Part model, mm, in its own coordinate system. A direction names the side the tool comes from. Round coordinates to 2 decimals unless told otherwise and drop trailing zeros. Write each loop counter-clockwise with the first axis right and the second up, starting at its lowest first coordinate (ties: lowest second). Pieces come first, ordered by that corner, then holes. Notation, with made-up numbers: M 63.5,84.5 L 117.5,84.5 A11 cw 117.5,89.5 Z; hole C 30,39.25 d11. An arc over 180 degrees is marked long. Answer as a JSON object with one key per item and string values. Group by question number.
1. Two-plate mould, pull along Z, no slides. Class faces 4 (the face through (-11.14, -28.26, -0.28)), 5 (the face through (-11, -27.52, 1)), 6 (the face through (-9.46, -29.85, -2.1)): +Z half, -Z half, draft (parallel to the pull), parting line (faces both ways), or undercut.
2. Band-saw the part on B-B, the plane y = -35. Write the cut outline in (x, z).
3. Band-saw the part on A-A, the plane z = 0. Write the cut outline in (x, y), plus the area to 3 significant figures.
4. Drop flat-ended pins along their axis: pin 1 (2 mm diameter, centred on x = -7, z = 1, fed in from -Y); pin 2 (2 mm diameter, centred on y = -34, z = 2.5, fed in from -X); pin 3 (1 mm diameter, centred on x = -12, y = -31, fed in from +Z). Give the stop position or say it passes through.
5. Which spindle directions (+Z, -Z, +X, -X, +Y, -Y) get a long thin tool onto all of the face, cutting with end or side? Do faces 1 (the face through (-11.77, -37.79, -0.77)), 2 (the face through (-10, -46, 0)), 3 (the face through (-10.78, -28.26, 0.91)). Say none if no direction does.
6. Drill centre lines: line 1 (Y direction, x = -12.5, z = -1.5); line 2 (X direction, y = -36.5, z = 1); line 3 (Y direction, x = -9.75, z = 2.25). Where is each one in solid material? Low to high. Write a range as from..to.
Autodesk Inventor part; units mm, degrees
ref_plane "YZ Plane" through (0, 0, 0) normal (1, 0, 0) x (0, 1, 0)
ref_plane "XZ Plane" through (0, 0, 0) normal (0, 1, 0) x (-1, 0, 0)
ref_plane "XY Plane" through (0, 0, 0) normal (0, 0, 1) x (1, 0, 0)
sketch "Sketch1" plane through (0, 0, 0) normal (0, 0, 1) x (1, 0, 0)
  line L0 (-14.4028, -27.52) -> (-9.9228, -27.52)
  line L1 (-9.9228, -27.52) -> (-9.9228, -31)
  line L2 (-9.9228, -31) -> (-9.9228, -46)
  line L3 (-9.9228, -46) -> (-11.9228, -46)
  line L4 (-11.9228, -46) -> (-11.9228, -30)
  line L5 (-11.9228, -30) -> (-14.4028, -27.52)
  line L6 (-11.9228, -30) -> (-6.9228, -30) construction
  point P0 (0, 0)
  dimension "d3" = 2
  dimension "d15" = 2.48
  dimension "d16" = 4.48
  dimension "d24" = 90
  dimension "d25" = 16
revolve "Revolution1" add sketch "Sketch1" angle 360 about axis through (-9.9228, -31, 0) along (0, -1, 0)
chamfer "Chamfer2" distance 0.2 angle 45 1 edges at (-7.9228, -46, 0)
thread "Rosca1"
chamfer "Chaflán3" distance 0.2 angle 45 1 edges at (-5.4428, -27.52, 0)
sketch "Boceto2" plane through (-9.9228, -27.52, 0) normal (0, 1, 0) x (1, 0, 0)
  line L0 (-1.0464, 0.9942) -> (0.3378, 1.4033)
  line L1 (0.3378, 1.4033) -> (1.3842, 0.4091)
  line L2 (1.3842, 0.4091) -> (1.0464, -0.9942)
  line L3 (1.0464, -0.9942) -> (-0.3378, -1.4033)
  line L4 (-0.3378, -1.4033) -> (-1.3842, -0.4091)
  line L5 (-1.3842, -0.4091) -> (-1.0464, 0.9942)
  point P0 (9.9228, 0)
  point P1 (0, 0)
  dimension "d20" = 2.5
extrude "Extrusión1" cut sketch "Boceto2" against normal blind 1.5
properties part number "Tornillo Allen cabeza fresada M4x16mm"
Worked answers:
{
 "1": {"face 4": "undercut", "face 5": "draft", "face 6": "parting line"},
 "2": {"outline": "C -9.92,0 d4"},
 "3": {"outline": "M -14.26,-27.66 L -11.92,-30 L -11.92,-45.8 L -11.72,-46 L -8.12,-46 L -7.92,-45.8 L -7.92,-30 L -5.58,-27.66 L -5.64,-27.52 L -8.64,-27.52 L -8.64,-29.02 L -11.21,-29.02 L -11.21,-27.52 L -14.2,-27.52 Z", "area": "76.1 mm^2"},
 "4": {"pin 1": "stops at y = -29.91", "pin 2": "stops at x = -11.25", "pin 3": "stops at z = 1.23"},
 "5": {"face 1": "-Y", "face 2": "+Z, -Z, +X, -X, -Y", "face 3": "+Y"},
 "6": {"line 1": "y = -29.02..-27.52", "line 2": "x = -11.65..-8.19", "line 3": "y = -29.74..-27.52"}
}
